Autodesk Inventor part; units mm, degrees
ref_plane "YZ Plane" through (0, 0, 0) normal (1, 0, 0) x (0, 1, 0)
ref_plane "XZ Plane" through (0, 0, 0) normal (0, 1, 0) x (-1, 0, 0)
ref_plane "XY Plane" through (0, 0, 0) normal (0, 0, 1) x (1, 0, 0)
sketch "Sketch1" plane through (0, 0, 0) normal (0, 0, 1) x (1, 0, 0)
  line L0 (0, 0) -> (-25, 0)
  line L1 (-25, 0) -> (-25, 100)
  line L2 (-25, 100) -> (0, 100)
  line L3 (0, 100) -> (0, 0)
  line L4 (0, 0) -> (-18, 0)
  line L5 (-18, 0) -> (-18, 85)
  line L6 (0, 85) -> (0, 0)
  line L7 (0, 85) -> (0, 65)
  line L8 (-18, 85) -> (-18, 100)
  point P0 (-18, 0)
  point P1 (-18, 92.5)
  dimension "d0" = 25
  dimension "d1" = 100
  dimension "d6" = 20
  dimension "d78" = 7
extrude "Extrusion1" add sketch "Sketch1" along normal blind 65 contours L0 L1 L2 L8 L5
sketch "Sketch2" plane through (-18, 0, 0) normal (1, 0, 0) x (0, 0, -1)
  line L0 (0, 0) -> (-65, 0)
  line L1 (0, 100) -> (-65, 100)
  line L2 (-47.5, 0) -> (-17.5, 0)
  line L3 (-17.5, 0) -> (-17.5, 100)
  line L4 (-17.5, 100) -> (-47.5, 100)
  line L5 (-47.5, 100) -> (-47.5, 0)
  line L6 (-65, 0) -> (-65, 100)
  line L7 (0, 0) -> (0, 100)
  line L8 (-47.5, 84.5192) -> (-17.5, 84.5192)
  dimension "d8" = 30
  dimension "d9" = 17.5
  dimension "d10" = 17.5
extrude "Extrusion2" add sketch "Sketch2" along normal blind 10 contours L0 L5 L8 L3
sketch "Sketch6" plane through (-8, 0, 0) normal (1, 0, 0) x (0, 0, -1)
  line L0 (0, 0) -> (-65, 0)
  line L1 (-60.5, 0) -> (-4.5, 0)
  line L2 (-4.5, 0) -> (-4.5, 85)
  line L3 (-4.5, 85) -> (-60.5, 85)
  line L4 (-60.5, 85) -> (-60.5, 0)
  line L5 (0, 0) -> (0, 100)
  line L6 (-65, 0) -> (-65, 100)
  line L7 (-57.5, 0) -> (-7.5, 0)
  line L8 (-7.5, 0) -> (-7.5, 82)
  line L9 (-7.5, 82) -> (-57.5, 82)
  line L10 (-57.5, 82) -> (-57.5, 0)
  line L11 (-57.5, 61) -> (-7.5, 61)
  line L12 (-57.5, 3) -> (-7.5, 3)
  point P0 (-32.5, 3)
  dimension "d27" = 56
  dimension "d28" = 85
  dimension "d29" = 4.5
  dimension "d30" = 4.5
  dimension "d31" = 50
  dimension "d32" = 3
  dimension "d33" = 3
  dimension "d34" = 61
  dimension "d49" = 3
hole "Hole3" at (-8, 61, 7.5) direction (-1, 0, 0) diameter 3 depth 40
hole "Hole4" at (-8, 82, 7.5) direction (-1, 0, 0) diameter 3 depth 40
hole "Hole5" at (-8, 3, 7.5) direction (-1, 0, 0) diameter 3 depth 40
hole "Hole6" at (-8, 3, 57.5) direction (-1, 0, 0) diameter 3 depth 40
hole "Hole7" at (-8, 61, 57.5) direction (-1, 0, 0) diameter 3 depth 40
hole "Hole8" at (-8, 82, 57.5) direction (-1, 0, 0) diameter 3 depth 40
fillet "Fillet1" radius 2 1 edges at (-8, 84.5192, 32.5)
properties part number "pi_holder"
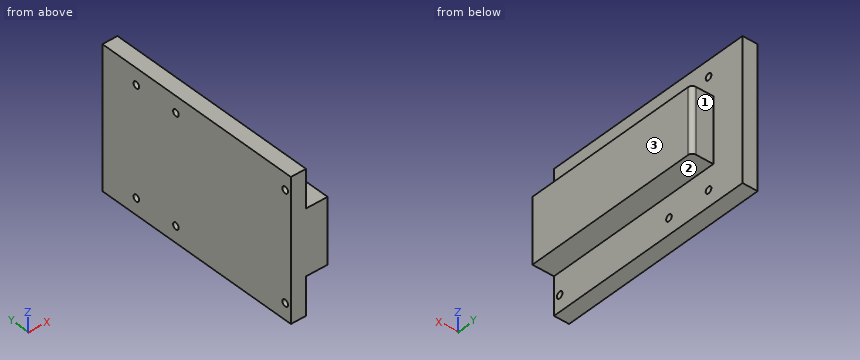
Part model, mm, in its own coordinate system. Face numbers are marked on the shaded views. A direction names the side the tool comes from. Round coordinates to 2 decimals unless told otherwise and drop trailing zeros. Write each loop counter-clockwise with the first axis right and the second up, starting at its lowest first coordinate (ties: lowest second). Pieces come first, ordered by that corner, then holes.
Item 1: Which spindle directions (+Z, -Z, +X, -X, +Y, -Y) get a long thin tool onto all of the face, cutting with end or side? Do the marked faces 1, 2 and 3. Say none if no direction does.
Results:
face 1: +Z, -Z, +X, +Y
face 2: -Z, +X, +Y, -Y
face 3: +Z, -Z, +X, +Y, -Y
Item 2: Drop flat-ended pins along their axis: pin 1 Ø2.5 at (x, z) = (-15, 38.5) entering from +Y; pin 2 Ø6 at (x, z) = (-18.5, 21.5) entering from -Y; pin 3 Ø5 at (x, y) = (-11, 34.5) entering from -Z; pin 4 Ø5 at (y, z) = (61, 57.5) entering from +X. Give the stop position or say it passes through.
Results:
pin 1: stops at y = 84.52
pin 2: stops at y = 0
pin 3: stops at z = 17.5
pin 4: stops at x = -18
Item 3: Cut at D-D, the plane y = 71.5. Give the cut face in (x, z), plus the area to 3 significant figures.
Results:
outline: (-25, 0) - (-18, 0) - (-18, 17.5) - (-8, 17.5) - (-8, 47.5) - (-18, 47.5) - (-18, 65) - (-25, 65) - close
area: 755 mm2
Item 4: Probe L1, parallel to Z at x = -23.25, y = 82; L2, parallel to Y at x = -20, z = 57.5; L3, parallel to Z at x = -15.25, y = 79. List the from-to ranges inside material, lowest first.
Results:
L1: z = 0 to 6, 9 to 56, 59 to 65
L2: y = 0 to 1.5, 4.5 to 59.5, 62.5 to 80.5, 83.5 to 100
L3: z = 17.5 to 47.5
Item 5: Cut at A-A, the plane y = 3. Give the cut face in (x, z), plus the area to 3 significant figures.
Results:
outline: (-25, 0) - (-18, 0) - (-18, 6) - (-25, 6) - close; (-25, 9) - (-18, 9) - (-18, 17.5) - (-8, 17.5) - (-8, 47.5) - (-18, 47.5) - (-18, 56) - (-25, 56) - close; (-25, 59) - (-18, 59) - (-18, 65) - (-25, 65) - close
area: 713 mm2
Item 6: Cut at C-C, the plane z = 28.5. Give the cut face in (x, y), plus the area to 3 significant figures.
Results:
outline: (-25, 0) - (-8, 0) - (-8, 82.52) arc R2 ccw to (-10, 84.52) - (-18, 84.52) - (-18, 100) - (-25, 100) - close
area: 1,540 mm2
Item 7: Cut at B-B, the plane z = 7.5. Give the cut face in (x, y).
Results:
outline: (-25, 0) - (-18, 0) - (-18, 1.5) - (-25, 1.5) - close; (-25, 4.5) - (-18, 4.5) - (-18, 59.5) - (-25, 59.5) - close; (-25, 62.5) - (-18, 62.5) - (-18, 80.5) - (-25, 80.5) - close; (-25, 83.5) - (-18, 83.5) - (-18, 100) - (-25, 100) - close
